Can you work these out from the model? Positions are in its coordinate system, mm. Coordinates: 2 decimals unless noted, no trailing zeros. Loops run counter-clockwise (first coordinate to the right, second up) from the corner with the lowest first, then second, coordinate; pieces in that order, holes last. Notation, with made-up numbers: (74, 31.5) - (86, 31.5) arc R16 ccw to (86, 47.5) - close; hole circle Ø1 at (80.25, 66.25). An arc over 180 degrees is marked (long way). Put each result on its own line as item: value. Start each with the question number.
Autodesk Fusion 360 part; units mm, degrees
sketch "Skizze1" plane through (0, 0, 0) normal (0, 0, 1) x (1, 0, 0)
  line L0 (0, 0) -> (21, 0)
  line L1 (21, 0) -> (21, 51)
  line L2 (21, 51) -> (0, 51)
  line L3 (0, 51) -> (0, 0)
  circle A0 centre (4.8, 49) radius 1.05
  circle A1 centre (16.2, 49) radius 1.05
  circle A2 centre (4.8, 2) radius 1.05
  circle A3 centre (16.2, 2) radius 1.05
  line L4 (6.5, 52.3) -> (14.5, 52.3)
  line L5 (14.5, 52.3) -> (14.5, 46.3)
  line L6 (14.5, 46.3) -> (6.5, 46.3)
  line L7 (6.5, 46.3) -> (6.5, 52.3)
  circle A4 centre (1.61, 49.63) radius 0.5
  circle A5 centre (19.39, 49.63) radius 0.5
  circle A6 centre (1.61, 47.09) radius 0.5
  circle A7 centre (19.39, 47.09) radius 0.5
  circle A8 centre (1.61, 44.55) radius 0.5
  circle A9 centre (19.39, 44.55) radius 0.5
  circle A10 centre (1.61, 42.01) radius 0.5
  circle A11 centre (19.39, 42.01) radius 0.5
  circle A12 centre (1.61, 39.47) radius 0.5
  circle A13 centre (19.39, 39.47) radius 0.5
  circle A14 centre (1.61, 36.93) radius 0.5
  circle A15 centre (19.39, 36.93) radius 0.5
  circle A16 centre (1.61, 34.39) radius 0.5
  circle A17 centre (19.39, 34.39) radius 0.5
  circle A18 centre (1.61, 31.85) radius 0.5
  circle A19 centre (19.39, 31.85) radius 0.5
  circle A20 centre (1.61, 29.31) radius 0.5
  circle A21 centre (19.39, 29.31) radius 0.5
  circle A22 centre (1.61, 26.77) radius 0.5
  circle A23 centre (19.39, 26.77) radius 0.5
  circle A24 centre (1.61, 24.23) radius 0.5
  circle A25 centre (19.39, 24.23) radius 0.5
  circle A26 centre (1.61, 21.69) radius 0.5
  circle A27 centre (19.39, 21.69) radius 0.5
  circle A28 centre (1.61, 19.15) radius 0.5
  circle A29 centre (19.39, 19.15) radius 0.5
  circle A30 centre (1.61, 16.61) radius 0.5
  circle A31 centre (19.39, 16.61) radius 0.5
  circle A32 centre (1.61, 14.07) radius 0.5
  circle A33 centre (19.39, 14.07) radius 0.5
  circle A34 centre (1.61, 11.53) radius 0.5
  circle A35 centre (19.39, 11.53) radius 0.5
  circle A36 centre (1.61, 8.99) radius 0.5
  circle A37 centre (19.39, 8.99) radius 0.5
  circle A38 centre (1.61, 6.45) radius 0.5
  circle A39 centre (19.39, 6.45) radius 0.5
  circle A40 centre (1.61, 3.91) radius 0.5
  circle A41 centre (19.39, 3.91) radius 0.5
  circle A42 centre (1.61, 1.37) radius 0.5
  circle A43 centre (19.39, 1.37) radius 0.5
  dimension "d1" = 21
  dimension "d2" = 51
  dimension "d3" = 2.1
  dimension "d4" = 4.8
  dimension "d5" = 2
  dimension "d8" = 11.4
  dimension "d9" = -47
  dimension "d10" = 8
  dimension "d11" = 6
  dimension "d12" = 1.3
  dimension "d13" = 6.5
  dimension "d20" = 1
  dimension "d21" = 1.37
  dimension "d22" = 1.61
  dimension "d25" = 17.78
  dimension "d26" = -2.54
extrude "Extrusion4" add sketch "Skizze1" along normal blind 1 contours L0 L1 L2 L3 L5 L6 L7
extrude "Extrusion2" add sketch "Skizze1" along normal blind 3.5 contours L2 L4 L5 L7 | L2 L5 L6 L7
extrude "Extrusion3" cut sketch "Skizze1" along normal blind 1 contours L2 L4 L5 L7
Q1. I want a section at C-C on x = 10.5. List the corners of the cut face in (y, z) for me.
Q2. I want a section at A-A on x = 16.2. List the corners of the cut face in (y, z) for me, and give its area (3 significant figures).
Q3. Will these pins go through, and if not, where does the flat tip stop? pin 1 (1 mm diameter, centred on x = 12.5, y = 34, fed in from -Z); pin 2 (1.2 mm diameter, centred on x = 9, z = 2.5, fed in from -Y); pin 3 (2.5 mm diameter, centred on x = 4.8, y = 2, fed in from +Z); pin 4 (1.4 mm diameter, centred on x = 10.5, y = 52, fed in from -Z).
Q4. We'd pull the mould along X, two halves only. Please class faces 1 (the flat face through (10.6, 51, 0.5)), 2 (the flat face through (6.5, 49, 2)), 3 (the cylindrical face through (19.3, 46.6, 0.5)): released by +X, released by -X, zero draft, split by the parting line, or undercut.
Q5. I want a section at D-D on x = 19.39. Count the separate pieces of the cut face and the enclosed holes in it, and give its area (3 significant figures).
Q6. I want a section at B-B on y = 8.99. List the corners of the cut face in (x, z) for me.
Q7. Please list where these lines run through material, in increasing order: line 1 along X through (y, z) = (42, 0.6); line 2 along Y through (x, z) = (15.5, 0.3); line 3 along Y through (x, z) = (17, 0.6). Write a range as [from, to].
Calculated:
1. outline: (0, 0) - (51, 0) - (51, 1) - (52.3, 1) - (52.3, 3.5) - (46.3, 3.5) - (46.3, 1) - (0, 1) - close
2. outline: (0, 0) - (0.95, 0) - (0.95, 1) - (0, 1) - close; (3.05, 0) - (47.95, 0) - (47.95, 1) - (3.05, 1) - close; (50.05, 0) - (51, 0) - (51, 1) - (50.05, 1) - close
2. area: 46.8 mm2
3. pin 1: z = 0
3. pin 2: y = 46.3
3. pin 3: z = 1
3. pin 4: z = 1
4. face 1: zero draft
4. face 2: released by -X
4. face 3: undercut
5. separate pieces: 21
5. enclosed holes: 0
5. area: 31.0 mm2
6. outline: (0, 0) - (1.11, 0) - (1.11, 1) - (0, 1) - close; (2.11, 0) - (18.89, 0) - (18.89, 1) - (2.11, 1) - close; (19.89, 0) - (21, 0) - (21, 1) - (19.89, 1) - close
7. line 1: [0, 1.11], [2.11, 18.89], [19.89, 21]
7. line 2: [0, 1.22], [2.78, 48.22], [49.78, 51]
7. line 3: [0, 1.32], [2.68, 48.32], [49.68, 51]
